from build123d import *

# Parameters (mm, degrees)
SKETCH1_W           = 118
SKETCH1_H           = 118
BOSS_EXTRUDE1_DEPTH = 15
SKETCH2_W           = 118
SKETCH2_H           = 118
SKETCH2_W_2         = 110
SKETCH2_H_2         = 110
CUT_EXTRUDE1_DEPTH  = 5
SKETCH6_R           = 69
BOSS_EXTRUDE2_DEPTH = 10
SKETCH3_R           = 52.5
CUT_EXTRUDE2_DEPTH  = 99.726896031
SKETCH4_R           = 65
CUT_EXTRUDE3_DEPTH  = 8
FILLET1_R           = 4
FILLET2_R           = 6.5


with BuildPart() as part:
    # Sketch1 → Boss-Extrude1 (new body)
    with BuildSketch(Plane(origin=(0, 0, 0), x_dir=(1, 0, 0), z_dir=(0, 1, 0))):
        Rectangle(SKETCH1_W, SKETCH1_H)
    extrude(amount=BOSS_EXTRUDE1_DEPTH)

    # Sketch2 → Cut-Extrude1 (cut)
    with BuildSketch(Plane.XZ):
        Rectangle(SKETCH2_W, SKETCH2_H)
        Rectangle(SKETCH2_W_2, SKETCH2_H_2, mode=Mode.SUBTRACT)
    extrude(amount=-CUT_EXTRUDE1_DEPTH, mode=Mode.SUBTRACT)

    # Sketch6 → Boss-Extrude2 (add)
    with BuildSketch(Plane(origin=(0, 15, 0), x_dir=(1, 0, 0), z_dir=(0, 1, 0))):
        Circle(SKETCH6_R)
    extrude(amount=-BOSS_EXTRUDE2_DEPTH)

    # Sketch3 → Cut-Extrude2 (cut, through all)
    with BuildSketch(Plane(origin=(0, 15, 0), x_dir=(1, 0, 0), z_dir=(0, 1, 0))):
        with Locations(Location((0, 0, 0), (0, 0, 270))):
            Circle(SKETCH3_R)
    extrude(amount=-CUT_EXTRUDE2_DEPTH, mode=Mode.SUBTRACT)

    # Sketch4 → Cut-Extrude3 (cut)
    with BuildSketch(Plane(origin=(0, 15, 0), x_dir=(1, 0, 0), z_dir=(0, 1, 0))):
        with Locations(Location((0, 0, 0), (0, 0, 270))):
            Circle(SKETCH4_R)
    extrude(amount=-CUT_EXTRUDE3_DEPTH, mode=Mode.SUBTRACT)

    # Fillet1
    fillet1_edges = [part.edges().sort_by_distance(p)[0] for p in [
        (55, 2.5, -55),
        (-55, 2.5, -55),
        (-55, 2.5, 55),
        (55, 2.5, 55),
    ]]
    fillet(fillet1_edges, radius=FILLET1_R)

    # Fillet2
    fillet2_edges = [part.edges().sort_by_distance(p)[0] for p in [
        (-59, 10, -59),
        (59, 10, -59),
        (59, 10, 59),
        (-59, 10, 59),
    ]]
    fillet(fillet2_edges, radius=FILLET2_R)


solid = part.part
Model file for the job. Use its own axes, mm. A direction names the side the tool comes from. Give positions to 0.01 mm unless a question says otherwise; leave off trailing zeros. Loops run counter-clockwise (first coordinate to the right, second up) from the corner with the lowest first, then second, coordinate; pieces in that order, holes last.
1) Flat gauge pins, fed straight in: pin 1 Ø3 at (x, y) = (42, 7.5) entering from -Z; pin 2 Ø4 at (y, z) = (5, -24) entering from -X; pin 3 Ø1.5 at (y, z) = (3.5, 11) entering from -X. Where does each tip first touch, or does it go through?
2) Saw through at D-D (y = 13). Write the cut outline in (x, z).
3) Saw through at A-A (x = 0). Write the cut outline in (y, z), plus the area to 3 significant figures.
4) Tool access for faces 5 (the cylindrical face through (-53.797, 2.535, 53.859)), 6 (the flat face through (44, 10, -59)), 7 (the flat face through (-44, 10, -59)): list every direction of +Z, -Z, +X, -X, +Y, -Y with a clear straight run to the whole face (end or side of a thin tool).
5) Saw through at C-C (z = 0). Write the cut outline in (x, y).
6) Saw through at B-B (y = 1.75). Write the cut outline in (x, z).
7) Wall check: line 1 (X direction, y = 3.75, z = 0); line 2 (Z direction, x = 34.5, y = 6.75); line 3 (Z direction, x = -21, y = 5.5). Give the ranges that are in metal, low to high.
8) Pull direction Z, two halves, no side cores. Call faces 1 (the cylindrical face through (-69, 10.1, -0.5)), 2 (the cylindrical face through (57.146, 10.07, -57.045)), 3 (the flat face through (-55, 2, -1)), 4 (the cylindrical face through (19.52, 11.06, 62)): +Z half, -Z half, draft (parallel to the pull), parting line (faces both ways), or undercut.
Answer block:
1. pin 1: stops at z = -59
1. pin 2: stops at x = -65.4
1. pin 3: stops at x = -55
2. outline: (-59, -52.5) arc R6.5 ccw to (-52.5, -59) - (-35.78, -59) arc R69 ccw to (35.78, -59) - (52.5, -59) arc R6.5 ccw to (59, -52.5) - (59, -35.78) arc R69 ccw to (59, 35.78) - (59, 52.5) arc R6.5 ccw to (52.5, 59) - (35.78, 59) arc R69 ccw to (-35.78, 59) - (-52.5, 59) arc R6.5 ccw to (-59, 52.5) - (-59, 35.78) arc R69 ccw to (-59, -35.78) - close; hole circle Ø130 at (0, 0)
3. outline: (0, -55) - (5, -55) - (5, -69) - (15, -69) - (15, -65) - (7, -65) - (7, -52.5) - (0, -52.5) - close; (0, 52.5) - (7, 52.5) - (7, 65) - (15, 65) - (15, 69) - (5, 69) - (5, 55) - (0, 55) - close
3. area: 155 mm2
4. face 5: +Z, -X, -Y
4. face 6: -Z, +X, +Y, -Y
4. face 7: -Z, -X, +Y, -Y
5. outline: (-69, 5) - (-55, 5) - (-55, 0) - (-52.5, 0) - (-52.5, 7) - (-65, 7) - (-65, 15) - (-69, 15) - close; (52.5, 0) - (55, 0) - (55, 5) - (69, 5) - (69, 15) - (65, 15) - (65, 7) - (52.5, 7) - close
6. outline: (-55, -51) arc R4 ccw to (-51, -55) - (51, -55) arc R4 ccw to (55, -51) - (55, 51) arc R4 ccw to (51, 55) - (-51, 55) arc R4 ccw to (-55, 51) - close; hole circle Ø105 at (0, 0)
7. line 1: x = -55 to -52.5, 52.5 to 55
7. line 2: z = -59.76 to -39.57, 39.57 to 59.76
7. line 3: z = -65.73 to -48.12, 48.12 to 65.73
8. face 1: parting line
8. face 2: -Z half
8. face 3: draft
8. face 4: undercut
